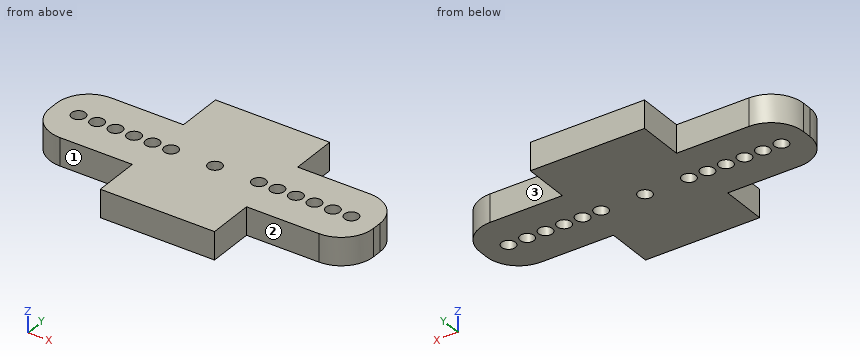
from build123d import *

# Parameters (mm, degrees)
SKETCH1_R           = 0.75
BOSS_EXTRUDE1_DEPTH = 1.5
SKETCH2_R           = 0.75
CUT_EXTRUDE1_DEPTH  = 4


with BuildPart() as part:
    # Sketch1 → Boss-Extrude1 (new body, symmetric)
    with BuildSketch(Plane.XY):
        with BuildLine():
            Line((-14, 4), (-6.175, 4))
            Line((-6.175, 4), (-6.175, 9))
            Line((-6.175, 9), (6.175, 9))
            Line((6.175, 9), (6.175, 4))
            Line((6.175, 4), (14, 4))
            ThreePointArc((14, 4), (16.474873734, 2.974873734), (17.5, 0.5))
            Line((17.5, 0.5), (17.5, -0.5))
            ThreePointArc((17.5, -0.5), (16.474873734, -2.974873734), (14, -4))
            Line((14, -4), (6.175, -4))
            Line((6.175, -4), (6.175, -9))
            Line((6.175, -9), (-6.175, -9))
            Line((-6.175, -9), (-6.175, -4))
            Line((-6.175, -4), (-14, -4))
            ThreePointArc((-14, -4), (-16.474873734, -2.974873734), (-17.5, -0.5))
            Line((-17.5, -0.5), (-17.5, 0.5))
            ThreePointArc((-17.5, 0.5), (-16.474873734, 2.974873734), (-14, 4))
        make_face()
        Circle(SKETCH1_R, mode=Mode.SUBTRACT)
    extrude(amount=BOSS_EXTRUDE1_DEPTH, both=True)

    # Sketch2 → Cut-Extrude1 (cut, through all)
    with BuildSketch(Plane.XY.offset(1.5)):
        with Locations((-14.75, 0)):
            Circle(SKETCH2_R)
        with Locations((-12.75, 0)):
            Circle(SKETCH2_R)
        with Locations((-10.75, 0)):
            Circle(SKETCH2_R)
        with Locations((-8.75, 0)):
            Circle(SKETCH2_R)
        with Locations((-6.75, 0)):
            Circle(SKETCH2_R)
        with Locations((-4.75, 0)):
            Circle(SKETCH2_R)
    cut_extrude1 = extrude(amount=-CUT_EXTRUDE1_DEPTH, mode=Mode.SUBTRACT)

    # Mirror1: Cut-Extrude1 across plane
    add(cut_extrude1.mirror(Plane(origin=(0, 0, 0), x_dir=(0, 0, 1), z_dir=(1, 0, 0))), mode=Mode.SUBTRACT)


solid = part.part
Source: CAD feature listing. Evaluate the final solid. Frame: model axes, mm. Face numbers are marked on the shaded views. A direction names the side the tool comes from. Round coordinates to 2 decimals unless told otherwise and drop trailing zeros. Loops run counter-clockwise (first coordinate to the right, second up) from the corner with the lowest first, then second, coordinate; pieces in that order, holes last.
Q1. First-contact query: P1, Ø0.9, axis at y = -7.5, z = 0, coming from the -X side (3 decimals); P2, Ø1.5, axis at y = 7.5, z = 0, coming from the +X side (3 decimals). Flat tips, straight axial feed; report the tip coordinate or a pass-through.
Q2. Access query for the marked faces 1, 2 and 3. Directions: +Z, -Z, +X, -X, +Y, -Y. A direction counts if a zero-diameter tool reaches every point of the face in a straight line with its end or side. Return the directions, or none.
Q3. Section C-C, the plane y = 7.75. Return loops of the section in (x, z) (3 decimals).
Q4. Ray query, line 1 (Y direction, x = -8.75, z = 0.5); line 2 (X direction, y = 7.5, z = 1.3) (3 decimals); line 3 (Y direction, x = -14.75, z = -0.1). Return the intervals inside material, ascending.
Q5. Section B-B, the plane z = 1. State how many separate pieces and enclosed holes the cut face has, plus the area to 3 significant figures.
Q6. Section A-A, the plane x = 4.75. Return loops of the section in (y, z), plus the area to 3 significant figures.
Solutions:
1. P1: stops at x = -6.175
1. P2: stops at x = 6.175
2. face 1: +Z, -Z, -X, -Y
2. face 2: +Z, -Z, +X, -Y
2. face 3: +Z, -Z, +X, +Y
3. outline: (-6.175, -1.5) - (6.175, -1.5) - (6.175, 1.5) - (-6.175, 1.5) - close
4. line 1: y = -4 to -0.75, 0.75 to 4
4. line 2: x = -6.175 to 6.175
4. line 3: y = -3.92 to -0.75, 0.75 to 3.92
5. separate pieces: 1
5. enclosed holes: 13
5. area: 370 mm2
6. outline: (-9, -1.5) - (-0.75, -1.5) - (-0.75, 1.5) - (-9, 1.5) - close; (0.75, -1.5) - (9, -1.5) - (9, 1.5) - (0.75, 1.5) - close
6. area: 49.5 mm2
